For this review, take the finished solid that the model builds, in its own axes (mm). Face numbers are marked on the shaded views. Coordinates: 2 decimals unless noted, no trailing zeros. Write each loop counter-clockwise with the first axis right and the second up, starting at its lowest first coordinate (ties: lowest second). Pieces come first, ordered by that corner, then holes.
1) We need section C-C on z = 174. Write out the cut boundary in (x, y).
2) We need section B-B on x = 42.5. Write out the cut boundary in (y, z), then the cut area to 3 significant figures.
3) Mouldability with a two-part tool opening along Z and no side actions: class the marked faces 1, 2, 3 and 4 as pulls with the +Z half, pulls with the -Z half, needs draft (parallel to the pull), parting line crosses it, or undercut.
4) We need section D-D on y = -55.5. Write out the cut boundary in (x, z).
5) To check wall thickness, follow line 1 along Z through (x, y) = (59, 11); line 2 along Y through (x, z) = (0, 86); line 3 along X through (y, z) = (3, 221). State the ranges of each line that lie inside material, in increasing order.
6) Insertion check: P1, Ø6, axis at y = 29.5, z = 65.5, coming from the -X side; P2, Ø7.5, axis at x = 34.9, y = -35.36, coming from the -Z side; P3, Ø3, axis at x = 23, z = 53.5, coming from the +Y side; P4, Ø4, axis at y = -17, z = 36, coming from the +X side. Each pin has a flat end and moves straight along its axis. Give the tip position at first contact, or say it passes through.
7) We need section A-A on y = 0. Write out the cut boundary in (x, z).
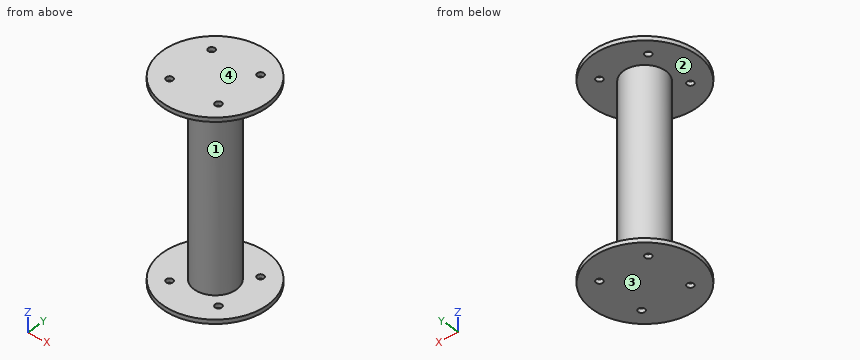
from build123d import *

# Parameters (mm, degrees)
F0_R     = 75
F0_R_2   = 4.7625
F1_DEPTH = 6
F2_R     = 30.15
F2_R_2   = 28.15
F3_DEPTH = 270
F5_R     = 75
F5_R_2   = 4.7625
F6_DEPTH = 6


with BuildPart() as f1:
    # F0 (on Top) → F1 (new body)
    with BuildSketch(Plane.XY):
        with Locations((-0.454545, 0)):
            Circle(F0_R)
        with Locations((-35.809885, -35.355339)):
            Circle(F0_R_2, mode=Mode.SUBTRACT)
        with Locations((34.900794, -35.355339)):
            Circle(F0_R_2, mode=Mode.SUBTRACT)
        with Locations((-35.809885, 35.355339)):
            Circle(F0_R_2, mode=Mode.SUBTRACT)
        with Locations((34.900794, 35.355339)):
            Circle(F0_R_2, mode=Mode.SUBTRACT)
    extrude(amount=F1_DEPTH)

    # F2 (on face) → F3 (join)
    with BuildSketch(Plane.XY.offset(6)):
        Circle(F2_R)
        Circle(F2_R_2, mode=Mode.SUBTRACT)
    extrude(amount=F3_DEPTH)

    # F5 (on offset) → F6 (join)
    with BuildSketch(Plane.XY.offset(276)):
        with Locations((-0.454545, 0)):
            Circle(F5_R)
        with Locations((-35.809885, -35.355339)):
            Circle(F5_R_2, mode=Mode.SUBTRACT)
        with Locations((34.900794, -35.355339)):
            Circle(F5_R_2, mode=Mode.SUBTRACT)
        with Locations((-35.809885, 35.355339)):
            Circle(F5_R_2, mode=Mode.SUBTRACT)
        with Locations((34.900794, 35.355339)):
            Circle(F5_R_2, mode=Mode.SUBTRACT)
    extrude(amount=F6_DEPTH)


solid = f1.part
Result:
1. outline: circle Ø60.3 at (0, 0); hole circle Ø56.3 at (0, 0)
2. outline: (-61.48, 0) - (61.48, 0) - (61.48, 6) - (-61.48, 6) - close; (-61.48, 276) - (61.48, 276) - (61.48, 282) - (-61.48, 282) - close
2. area: 1,480 mm2
3. face 1: undercut
3. face 2: undercut
3. face 3: pulls with the -Z half
3. face 4: pulls with the +Z half
4. outline: (-50.9, 0) - (49.99, 0) - (49.99, 6) - (-50.9, 6) - close; (-50.9, 276) - (49.99, 276) - (49.99, 282) - (-50.9, 282) - close
5. line 1: z = 0 to 6, 276 to 282
5. line 2: y = -30.15 to -28.15, 28.15 to 30.15
5. line 3: x = -30 to -27.99, 27.99 to 30
6. P1: stops at x = -14.38
6. P2: passes through
6. P3: stops at y = 21.14
6. P4: stops at x = 26.15
7. outline: (-75.45, 0) - (74.55, 0) - (74.55, 6) - (30.15, 6) - (30.15, 276) - (74.55, 276) - (74.55, 282) - (-75.45, 282) - (-75.45, 276) - (-30.15, 276) - (-30.15, 6) - (-75.45, 6) - close; hole (-28.15, 6) - (28.15, 6) - (28.15, 276) - (-28.15, 276) - close
